from build123d import *

# Parameters (mm, degrees)
SKETCH_1_W             = 34
SKETCH_1_H             = 34
SKETCH_1_R             = 13
EXTRUDE_1_DEPTH        = 48
SKETCH_2_R             = 13.5
CUT_EXTRUDE_1_DEPTH    = 10
SKETCH_3_R             = 13
CUT_EXTRUDE_2_DEPTH    = 10
CHAMFER_1_SIZE         = 10
CHAMFER_2_SIZE         = 28
SKETCH_5_R             = 16
CUT_EXTRUDE_4_DEPTH    = 14
HOLE_WIZARD_M4_1_D     = 3.3
HOLE_WIZARD_M4_1_DEPTH = 8
HOLE_WIZARD_M4_1_TIP   = 0.991420021
SKETCH_8_W             = 1.3
SKETCH_8_H             = 1.5


with BuildPart() as part:
    # 草图1 → 凸台-拉伸1 (new body)
    with BuildSketch(Plane.XY):
        Rectangle(SKETCH_1_W, SKETCH_1_H)
        Circle(SKETCH_1_R, mode=Mode.SUBTRACT)
    extrude(amount=EXTRUDE_1_DEPTH)

    # 草图2 → 切除-拉伸1 (cut)
    with BuildSketch(Plane.XY.offset(48)):
        Circle(SKETCH_2_R)
    extrude(amount=-CUT_EXTRUDE_1_DEPTH, mode=Mode.SUBTRACT)

    # 草图3 → 切除-拉伸2 (cut)
    with BuildSketch(Plane.XZ.offset(17)):
        with Locations(Location((0, 17, 0), (0, 0, 270))):
            Circle(SKETCH_3_R)
    extrude(amount=-CUT_EXTRUDE_2_DEPTH, mode=Mode.SUBTRACT)

    # 倒角1
    chamfer_1_edges = [part.edges().sort_by_distance(p)[0] for p in [
        (-17, 17, 24),
        (17, 17, 24),
    ]]
    chamfer(chamfer_1_edges, length=CHAMFER_1_SIZE)

    # 倒角2
    # the kernel refuses this chamfer: 28 mm, written as the material it takes off along each edge
    with BuildSketch(Plane(origin=(79.007123663, 17, 0), x_dir=(0, -0.9996219169112968, -0.027495876610586376), z_dir=(-1, 0, 0))) as chamfer_2_piece_1:
        Polygon((CHAMFER_2_SIZE * 0.999621916911, CHAMFER_2_SIZE * 0.0274958766106), (-CHAMFER_2_SIZE * 0.0274958766106, CHAMFER_2_SIZE * 0.999621916911), (0, 0), align=None)
    extrude(amount=158.014247326, mode=Mode.SUBTRACT)

    # 草图5 → 切除-拉伸4 (cut)
    with BuildSketch(Plane.XY.offset(48)):
        Polygon((-7, 17), (-17, 7), (-17, -17), (17, -17), (17, 7), (7, 17), align=None)
        Circle(SKETCH_5_R, mode=Mode.SUBTRACT)
    extrude(amount=-CUT_EXTRUDE_4_DEPTH, mode=Mode.SUBTRACT)

    # M4 螺纹孔1
    with Locations(Plane.XZ.offset(17)):
        with Locations((13, 30), (13, 4), (-13, 4), (-13, 30)):
            Hole(HOLE_WIZARD_M4_1_D / 2, depth=HOLE_WIZARD_M4_1_DEPTH)
            with Locations((0, 0, -(HOLE_WIZARD_M4_1_DEPTH + HOLE_WIZARD_M4_1_TIP / 2))):  # 118° drill point
                Cone(0, HOLE_WIZARD_M4_1_D / 2, HOLE_WIZARD_M4_1_TIP, mode=Mode.SUBTRACT)

    # 草图8 → 切除-旋转1 (revolve, cut)
    with BuildSketch(Plane(origin=(0, 0, 0), x_dir=(0, 0, -1), z_dir=(1, 0, 0)), mode=Mode.PRIVATE) as cut_revolve_1_sk:
        with Locations((-46.65, 14.25)):
            Rectangle(SKETCH_8_W, SKETCH_8_H)
    revolve(cut_revolve_1_sk.sketch.rotate(Axis((0, 0, 0), (0, 0, 1)), 147.795772496), axis=Axis((0, 0, 0), (0, 0, 1)), mode=Mode.SUBTRACT)


solid = part.part
Part model, mm, in its own coordinate system. A direction names the side the tool comes from. Coordinates: 2 decimals unless noted, no trailing zeros. Order: outer loops, then holes, each group sorted by start corner. A loop starts at its lowest first (then second) coordinate and runs counter-clockwise, first axis right, second up. Notation, with made-up numbers: M 3,-5 L 34,-5 A22 ccw 34,5 Z; hole C 10,65.25 d6. An arc over 180 degrees is marked long. Use a Markdown table: item, result.
(1) Flat gauge pins, fed straight in: pin 1 (15 mm diameter, centred on x = -4.5, y = -4.5, fed in from -Z); pin 2 (5 mm diameter, centred on y = -3, z = 40.5, fed in from +X); pin 3 (15.5 mm diameter, centred on x = 0, z = 17, fed in from +Y); pin 4 (10 mm diameter, centred on x = 11.5, z = 18, fed in from +Y). Where does each tip first touch, or does it go through?
A:
| item | result |
|---|---|
| pin 1 | stops at z = 0 |
| pin 2 | stops at x = 15.99 |
| pin 3 | stops at y = 13.75 |
| pin 4 | stops at y = 12 |
(2) Probe L1, parallel to Y at x = -0.5, z = 41; L2, parallel to X at y = -9.25, z = 17. List the from-to ranges inside material, lowest first.
A:
| item | result |
|---|---|
| L1 | y = -15.99 to -13.49, 13.49 to 15.99 |
| L2 | x = -17 to -13, 13 to 17 |
(3) Pull direction Y, two halves, no side cores. Call faces 6 (the conical face through (-13.23, -8.18, 29.83)), 7 (the cylindrical face through (-3.47, -15.62, 41.1)), 8 (the flat face through (-5, -13, 46)): released by +Y, released by -Y, zero draft, split by the parting line, or undercut.
A:
| item | result |
|---|---|
| face 6 | released by -Y |
| face 7 | split by the parting line |
| face 8 | undercut |
(4) Cut at D-D on x = 6. Write the cut outline in (y, z), then the cut area to 3 significant figures.
A:
| item | result |
|---|---|
| outline | M -17,0 L -11.53,0 L -11.53,5.47 L -17,5.47 Z; M -17,28.53 L -11.53,28.53 L -11.53,38 L -12.09,38 L -12.09,46 L -13.75,46 L -13.75,47.3 L -12.09,47.3 L -12.09,48 L -14.83,48 L -14.83,34 L -17,34 Z; M 11.53,22.53 L 17,28 L 17,34 L 14.83,34 L 14.83,48 L 12.09,48 L 12.09,47.3 L 13.75,47.3 L 13.75,46 L 12.09,46 L 12.09,38 L 11.53,38 Z |
| area | 184 mm^2 |
(5) Cut at A-A on x = -4. Write the cut outline in (y, z), then the cut area to 3 significant figures.
A:
| item | result |
|---|---|
| outline | M -17,0 L -12.37,0 L -12.37,4.63 L -17,4.63 Z; M -17,29.37 L -12.37,29.37 L -12.37,38 L -12.89,38 L -12.89,46 L -14.46,46 L -14.46,47.3 L -12.89,47.3 L -12.89,48 L -15.49,48 L -15.49,34 L -17,34 Z; M 12.37,23.37 L 17,28 L 17,34 L 15.49,34 L 15.49,48 L 12.89,48 L 12.89,47.3 L 14.46,47.3 L 14.46,46 L 12.89,46 L 12.89,38 L 12.37,38 Z |
| area | 154 mm^2 |
(6) Cut at C-C on z = 21. Write the cut outline in (x, y), then the cut area to 3 significant figures.
A:
| item | result |
|---|---|
| outline | M -17,-17 L -12.37,-17 L -12.37,-7 L -10.95,-7 A13 cw -8.31,10 L -14,10 L -17,7 Z; M 8.31,10 A13 cw 10.95,-7 L 12.37,-7 L 12.37,-17 L 17,-17 L 17,7 L 14,10 Z |
| area | 257 mm^2 |
(7) Tool access for faces 1 (the flat face through (17, -8, 21)), 2 (the flat face through (13, 11, 28)), 3 (the cylindrical face through (-12, -9, 47)), 4 (the cylindrical face through (3.9, -13.2, 4.6)), 5 (the cylindrical face through (12.877, 4.055, 42.056)): list every direction of +Z, -Z, +X, -X, +Y, -Y with a clear straight run to the whole face (end or side of a thin tool).
A:
| item | result |
|---|---|
| face 1 | +Z, -Z, +X, +Y, -Y |
| face 2 | +Z, -Z, +X, +Y |
| face 3 | none |
| face 4 | -Y |
| face 5 | +Z |
(8) Cut at B-B on y = 4. Write the cut outline in (x, z), then the cut area to 3 significant figures.
A:
| item | result |
|---|---|
| outline | M -17,15 L -12.37,15 L -12.37,38 L -12.89,38 L -12.89,46 L -14.46,46 L -14.46,47.3 L -12.89,47.3 L -12.89,48 L -15.49,48 L -15.49,34 L -17,34 Z; M 12.37,15 L 17,15 L 17,34 L 15.49,34 L 15.49,48 L 12.89,48 L 12.89,47.3 L 14.46,47.3 L 14.46,46 L 12.89,46 L 12.89,38 L 12.37,38 Z |
| area | 249 mm^2 |
